Read the model definition and answer for the solid it produces. Units are mm, in the model's axes. Face numbers are marked on the shaded views. A direction names the side the tool comes from. Round coordinates to 2 decimals unless told otherwise and drop trailing zeros. Order: outer loops, then holes, each group sorted by start corner. A loop starts at its lowest first (then second) coordinate and runs counter-clockwise, first axis right, second up. Notation, with made-up numbers: (78.25, 68) -> (117.25, 68) arc R18 cw to (117.25, 77) -> close; hole circle Ø2 at (-39.5, 74). An arc over 180 degrees is marked (long way). Answer as a JSON object with one key per item and string values. Group by question number.
Item 1: Section A-A, the plane z = 0 is taken. Write down the section's boundary in (x, y) (3 decimals).
Item 2: Consider probe 1 along Z at (x, y) = (-0.1, 14.5); probe 2 along Z at (x, y) = (2.45, 28); probe 3 along Y at (x, z) = (-1.6, -1.6). Determine where each line is inside the solid, lowest interval first. Write a range as from..to.
Item 3: Given P1, Ø1.5, axis at x = -1.5, y = 14, coming from the +Z side; P2, Ø2, axis at y = 27, z = 2, coming from the -X side; P3, Ø2, axis at x = -1, z = 2.5, coming from the +Y side, each flat-ended and moving along its own axis, determine where each tip first touches the part or whether it passes through.
Item 4: Section B-B, the plane x = 0 is taken. Write down the section's boundary in (y, z) (3 decimals).
Item 5: For the marked faces 1 and 2, determine the directions among +Z, -Z, +X, -X, +Y, -Y from which every point of the face is accessible in a straight line to the end or side of a thin tool.
Item 6: Section C-C, the plane y = 36.5 is taken. Write down the section's boundary in (x, z), plus the area to 3 significant figures.
Autodesk Inventor part; units mm, degrees
ref_plane "YZ Plane" through (0, 0, 0) normal (1, 0, 0) x (0, 1, 0)
ref_plane "XZ Plane" through (0, 0, 0) normal (0, 1, 0) x (-1, 0, 0)
ref_plane "XY Plane" through (0, 0, 0) normal (0, 0, 1) x (1, 0, 0)
sketch "Sketch1" plane through (0, 0, 0) normal (0, 0, 1) x (1, 0, 0)
  line L0 (-3.6, 0) -> (0.6, 0) construction
  line L1 (0, 0) -> (-3, 0)
  line L2 (-3, 0) -> (-3, 38.8)
  line L3 (-3, 38.8) -> (-1.725, 41.0084)
  line L4 (-1.725, 41.0084) -> (-1.725, 51.425)
  line L5 (-1.725, 51.425) -> (-1.15, 52)
  line L6 (-1.15, 52) -> (-1.15, 57)
  line L7 (-1.15, 57) -> (0, 57)
  line L8 (0, 57) -> (0, 0)
  dimension "d0" = 57
  dimension "d10" = 5
  dimension "d13" = 5.575
  dimension "d16" = 38.8
  dimension "d17" = 6
  dimension "d18" = 3.45
  dimension "d19" = 2.3
  dimension "d20" = 30
  dimension "d21" = 45
revolve "Revolution1" add sketch "Sketch1" angle 360 about axis through (0, 57, 0) along (0, -1, 0)
properties part number "R217.13-023050CC06K 1630"
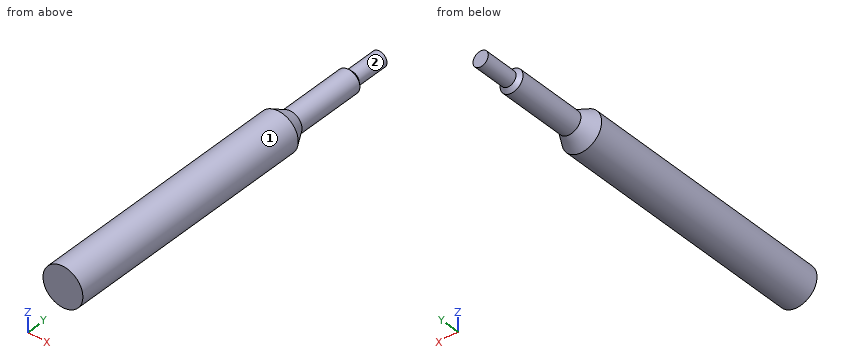
Values found:
{
 "1": {"outline": "(-3, 0) -> (3, 0) -> (3, 38.8) -> (1.725, 41.008) -> (1.725, 51.425) -> (1.15, 52) -> (1.15, 57) -> (-1.15, 57) -> (-1.15, 52) -> (-1.725, 51.425) -> (-1.725, 41.008) -> (-3, 38.8) -> close"},
 "2": {"probe 1": "-3..3", "probe 2": "-1.73..1.73", "probe 3": "0..40.08"},
 "3": {"P1": "z = 2.9", "P2": "x = -2.83", "P3": "y = 51.46"},
 "4": {"outline": "(0, -3) -> (38.8, -3) -> (41.008, -1.725) -> (51.425, -1.725) -> (52, -1.15) -> (57, -1.15) -> (57, 1.15) -> (52, 1.15) -> (51.425, 1.725) -> (41.008, 1.725) -> (38.8, 3) -> (0, 3) -> close"},
 "5": {"face 1": "+Y, -Y", "face 2": "+Y"},
 "6": {"outline": "circle Ø6 at (0, 0)", "area": "28.3 mm2"}
}
